from build123d import *

# Parameters (mm, degrees)
SKETCH1_W           = 231.14
SKETCH1_H           = 162.56
BOSS_EXTRUDE1_DEPTH = 5.08
SKETCH2_R           = 1.37795
CUT_EXTRUDE1_DEPTH  = 142.381291902
CAVITY2_START       = -81.28
CAVITY2_OUTLINE_W   = 77.046666667
CAVITY2_OUTLINE_H   = 5.08
CAVITY2_DEPTH       = 5.08
CAVITY2_START_2     = 76.2
CAVITY2_2_OUTLINE_W = 77.046666667
CAVITY2_2_OUTLINE_H = 5.08
CAVITY2_2_DEPTH     = 5.08
CAVITY2_START_3     = -76.2
CAVITY2_3_OUTLINE_W = 5.08
CAVITY2_3_OUTLINE_H = 5.08
CAVITY2_3_DEPTH     = 49.106666667
CAVITY2_START_4     = 27.093333333
CAVITY2_4_OUTLINE_W = 5.08
CAVITY2_4_OUTLINE_H = 5.08
CAVITY2_4_DEPTH     = 49.106666667
SKETCH3_W           = 15.748
SKETCH3_H           = 7.112
CUT_EXTRUDE2_DEPTH  = 142.381291902


# Read off the part's stored shape, not the designer's step: Cavity2
with BuildPart() as part:
    # Sketch1 → Boss-Extrude1 (new body)
    with BuildSketch(Plane.XY):
        Rectangle(SKETCH1_W, SKETCH1_H)
    extrude(amount=BOSS_EXTRUDE1_DEPTH)

    # Sketch2 → Cut-Extrude1 (cut, through all)
    with BuildSketch(Plane(origin=(0, 0, 0), x_dir=(-1, 0, 0), z_dir=(0, 0, -1))):
        with Locations((-113.03, 0)):
            Circle(SKETCH2_R)
        with Locations(Location((0, 78.74, 0), (0, 0, 180))):
            Circle(SKETCH2_R)
        with Locations(Location((113.03, 0, 0), (0, 0, 180))):
            Circle(SKETCH2_R)
        with Locations((0, -78.74)):
            Circle(SKETCH2_R)
    extrude(amount=-CUT_EXTRUDE1_DEPTH, mode=Mode.SUBTRACT)

    # Cavity2 outline → Cavity2 (cut)
    with BuildSketch(Plane(origin=(0, 0, 0), x_dir=(1, 0, 0), z_dir=(0, 1, 0)).offset(CAVITY2_START)):
        with Locations((-77.046666667, -2.54)):
            Rectangle(CAVITY2_OUTLINE_W, CAVITY2_OUTLINE_H)
        with Locations((77.046666667, -2.54)):
            Rectangle(CAVITY2_OUTLINE_W, CAVITY2_OUTLINE_H)
    extrude(amount=CAVITY2_DEPTH, mode=Mode.SUBTRACT)

    # Cavity2 2 outline → Cavity2 2 (cut)
    with BuildSketch(Plane(origin=(0, 0, 0), x_dir=(1, 0, 0), z_dir=(0, 1, 0)).offset(CAVITY2_START_2)):
        with Locations((-77.046666667, -2.54)):
            Rectangle(CAVITY2_2_OUTLINE_W, CAVITY2_2_OUTLINE_H)
        with Locations((77.046666667, -2.54)):
            Rectangle(CAVITY2_2_OUTLINE_W, CAVITY2_2_OUTLINE_H)
    extrude(amount=CAVITY2_2_DEPTH, mode=Mode.SUBTRACT)

    # Cavity2 3 outline → Cavity2 3 (cut)
    with BuildSketch(Plane(origin=(0, 0, 0), x_dir=(1, 0, 0), z_dir=(0, 1, 0)).offset(CAVITY2_START_3)):
        with Locations((-113.03, -2.54)):
            Rectangle(CAVITY2_3_OUTLINE_W, CAVITY2_3_OUTLINE_H)
        with Locations((113.03, -2.54)):
            Rectangle(CAVITY2_3_OUTLINE_W, CAVITY2_3_OUTLINE_H)
    extrude(amount=CAVITY2_3_DEPTH, mode=Mode.SUBTRACT)

    # Cavity2 4 outline → Cavity2 4 (cut)
    with BuildSketch(Plane(origin=(0, 0, 0), x_dir=(1, 0, 0), z_dir=(0, 1, 0)).offset(CAVITY2_START_4)):
        with Locations((-113.03, -2.54)):
            Rectangle(CAVITY2_4_OUTLINE_W, CAVITY2_4_OUTLINE_H)
        with Locations((113.03, -2.54)):
            Rectangle(CAVITY2_4_OUTLINE_W, CAVITY2_4_OUTLINE_H)
    extrude(amount=CAVITY2_4_DEPTH, mode=Mode.SUBTRACT)

    # Sketch3 → Cut-Extrude2 (cut, through all)
    with BuildSketch(Plane(origin=(0, 0, 0), x_dir=(-1, 0, 0), z_dir=(0, 0, -1))):
        with Locations((83.82, 49.53)):
            Rectangle(SKETCH3_W, SKETCH3_H)
    extrude(amount=-CUT_EXTRUDE2_DEPTH, mode=Mode.SUBTRACT)


solid = part.part
Could you check a few things on this model? Use its own coordinates, in mm. A direction names the side the tool comes from. Give positions to 0.01 mm unless a question says otherwise; leave off trailing zeros. Loops run counter-clockwise (first coordinate to the right, second up) from the corner with the lowest first, then second, coordinate; pieces in that order, holes last. Notation, with made-up numbers: (64.25, -27.75) -> (117.25, -27.75) arc R34 ccw to (117.25, 8.25) -> close; hole circle Ø4 at (44.5, -4.5). An arc over 180 degrees is marked (long way). Return JSON: item names as keys, results as strings.
Item 1: If we section it at A-A on y = -59: List the corners of the cut face in (x, z) for me.
Geometry results:
{"outline": "(-110.49, 0) -> (110.49, 0) -> (110.49, 5.08) -> (-110.49, 5.08) -> close"}
Item 2: If we section it at B-B on x = -49.5: List the corners of the cut face in (y, z) for me.
Geometry results:
{"outline": "(-76.2, 0) -> (76.2, 0) -> (76.2, 5.08) -> (-76.2, 5.08) -> close"}
Item 3: I need wall thicknesses on L1, parallel to Y at x = 0, z = 2.8; L2, parallel to Y at x = -113.03, z = 3.3; L3, parallel to X at y = 78.74, z = 2.75. Which ranges of each line are inside material? Lowest first, please. Write a range as from..to.
Geometry results:
{"L1": "y = -81.28..-80.12, -77.36..77.36, 80.12..81.28", "L2": "y = -27.09..-1.38, 1.38..27.09", "L3": "x = -38.52..-1.38, 1.38..38.52"}
Item 4: Which directions (+Z, -Z, +X, -X, +Y, -Y) give clear straight access to the entire face, cutting with the end or side of a thin tool? Please do faces 1 (the flat face through (-113, 27.093, 3)), 2 (the flat face through (-84, 45.974, 3)), 3 (the flat face through (113, -27.093, 3)), 4 (the flat face through (110.49, 51, 3)).
Geometry results:
{"face 1": "+Z, -Z, -X, +Y", "face 2": "+Z, -Z", "face 3": "+Z, -Z, +X, -Y", "face 4": "+Z, -Z, +X, +Y"}
Item 5: I'm going to push flat-ended pins straight in: pin 1 (2.5 mm diameter, centred on y = 48.5, z = 1.5, fed in from -X); pin 2 (1.5 mm diameter, centred on x = -85, z = 3, fed in from +Y); pin 3 (2 mm diameter, centred on x = 66.5, z = 1.5, fed in from -Y). Where does each tip first touch, or does it pass through?
Geometry results:
{"pin 1": "stops at x = -110.49", "pin 2": "stops at y = 76.2", "pin 3": "stops at y = -76.2"}
